Verification items for the finished model (mm, model axes). A direction names the side the tool comes from. Coordinates: 2 decimals unless noted, no trailing zeros. Write each loop counter-clockwise with the first axis right and the second up, starting at its lowest first coordinate (ties: lowest second). Pieces come first, ordered by that corner, then holes. Notation, with made-up numbers: (56.25, 10) - (60.25, 10) arc R23 ccw to (60.25, 22) - close; hole circle Ø2 at (35, 87). An arc over 180 degrees is marked (long way). Use one line per item in the form item = value. Start each with the question number.
(1) Tool access check on faces 1 (the cylindrical face through (-290.61, 3, 30.54)), 2 (the cylindrical face through (-283, 0, 7)), 3 (the flat face through (-3, 0, 42)), 4 (the flat face through (-290, 20.5, 21)). Record the directions out of +Z, -Z, +X, -X, +Y, -Y that give a thin tool (end or side, any length) a straight path to the whole face; none if there is none.
(2) Gauge pin test, flat ends, axial feed: pin 1 Ø5 at (x, y) = (-348.5, 14.5) entering from -Z; pin 2 Ø6 at (x, z) = (-383, 20.5) entering from -Y; pin 3 Ø6 at (x, z) = (-38.5, 31) entering from -Y. Record the tip position at first contact, or that the pin passes through.
(3) Mould release check, pull along Y, two halves, no side actions. Record for faces 5 (the cylindrical face through (-283, 0, 35)), 6 (the flat face through (-545, 10.2, 20.8)), 7 (the flat face through (-29, 0, 21)), 8 (the flat face through (-3, -21, 21)): released by +Y, released by -Y, zero draft, split by the parting line, or undercut.
(4) Sectioned sample at A-A (y = 0). Record the cut outline in (x, z), and give its area (3 significant figures).
(5) Material ranges on line 1 (Y direction, x = -67, z = 29); line 2 (Z direction, x = -509, y = 12.5); line 3 (Y direction, x = -13, z = 24), recorded low to high. Write a range as [from, to].
from build123d import *

# Parameters (mm, degrees)
SKETCH_1_W          = 516
SKETCH_1_H          = 35
SKETCH_1_W_2        = 5
SKETCH_1_H_2        = 42
SKETCH_1_W_3        = 48
EXTRUDE_1_DEPTH     = 42
SKETCH_3_W          = 516
SKETCH_3_H          = 42
CUT_EXTRUDE_1_DEPTH = 0.5
FILLET_1_R          = 7
SKETCH_4_R          = 10
CUT_EXTRUDE_2_DEPTH = 516
CUT_EXTRUDE_START   = -516
CUT_EXTRUDE_3_DEPTH = 516
FILLET_2_R          = 2
FILLET_3_R          = 4
FILLET_5_R          = 1
SKETCH_6_W          = 6.5
SKETCH_6_H          = 16
EXTRUDE_2_DEPTH     = 8


# Read off the part's stored shape, not the designer's step: Вырез-Вытянуть3
with BuildPart() as part:
    # Эскиз1 → Бобышка-Вытянуть1 (new body)
    with BuildSketch(Plane.XY):
        with Locations((-287, 3.5)):
            Rectangle(SKETCH_1_W, SKETCH_1_H)
        with Locations((-26.5, 0)):
            Rectangle(SKETCH_1_W_2, SKETCH_1_H_2)
        Rectangle(SKETCH_1_W_3, SKETCH_1_H_2)
    extrude(amount=EXTRUDE_1_DEPTH)

    # Эскиз3 → Вырез-Вытянуть1 (cut)
    with BuildSketch(Plane(origin=(0, 21, 0), x_dir=(1, 0, 0), z_dir=(0, 1, 0))):
        with Locations((-287, -21)):
            Rectangle(SKETCH_3_W, SKETCH_3_H)
    extrude(amount=-CUT_EXTRUDE_1_DEPTH, mode=Mode.SUBTRACT)

    # Скругление1
    fillet_1_edges = [part.edges().sort_by_distance(p)[0] for p in [
        (-287, -14, 42),
        (-287, -14, 0),
        (-287, 20.5, 0),
        (-287, 20.5, 42),
    ]]
    fillet(fillet_1_edges, radius=FILLET_1_R)

    # Эскиз4 → Вырез-Вытянуть2 (cut)
    with BuildSketch(Plane.ZY.offset(545)):
        with Locations((21, 0)):
            Circle(SKETCH_4_R)
    extrude(amount=-CUT_EXTRUDE_2_DEPTH, mode=Mode.SUBTRACT)

    # Вырез-Вытянуть3 outline → Вырез-Вытянуть3 (cut)
    with BuildSketch(Plane.ZY.offset(545).offset(CUT_EXTRUDE_START)):
        with BuildLine():
            ThreePointArc((11.715680056, -10.478616473), (8.035714286, -10.206727973), (8.63508525, -6.565735543))
            ThreePointArc((8.63508525, -6.565735543), (7, 0), (8.63508525, 6.565735543))
            ThreePointArc((8.63508525, 6.565735543), (7.60351338, 9.372189345), (10, 11.160254038))
            Line((10, 11.160254038), (10, 20.5))
            Line((10, 20.5), (7, 20.5))
            ThreePointArc((7, 20.5), (2.050252532, 18.449747468), (0, 13.5))
            Line((0, 13.5), (0, -7))
            ThreePointArc((0, -7), (2.050252532, -11.949747468), (7, -14))
            Line((7, -14), (21.000000051, -14))
            ThreePointArc((21.000000051, -14), (16.035155143, -13.090084627), (11.715680056, -10.478616473))
        make_face()
        with BuildLine():
            ThreePointArc((30.284319944, -10.478616473), (25.964844905, -13.090084609), (21.000000051, -14))
            Line((21.000000051, -14), (35, -14))
            ThreePointArc((35, -14), (39.949747468, -11.949747468), (42, -7))
            Line((42, -7), (42, 13.5))
            ThreePointArc((42, 13.5), (39.949747468, 18.449747468), (35, 20.5))
            Line((35, 20.5), (32, 20.5))
            Line((32, 20.5), (32, 11.160254038))
            ThreePointArc((32, 11.160254038), (34.39648662, 9.372189345), (33.36491475, 6.565735543))
            ThreePointArc((33.36491475, 6.565735543), (35, 0), (33.36491475, -6.565735543))
            ThreePointArc((33.36491475, -6.565735543), (33.964285714, -10.206727973), (30.284319944, -10.478616473))
        make_face()
    extrude(amount=CUT_EXTRUDE_3_DEPTH, mode=Mode.SUBTRACT)

    # Скругление2
    fillet_2_edges = [part.edges().sort_by_distance(p)[0] for p in [
        (-287, 20.5, 10),
        (-287, 20.5, 32),
    ]]
    fillet(fillet_2_edges, radius=FILLET_2_R)

    # Скругление3
    fillet_3_edges = [part.edges().sort_by_distance(p)[0] for p in [
        (-2.5, -21, 42),
        (-2.5, 21, 42),
        (-2.5, 21, 0),
        (-2.5, -21, 0),
    ]]
    fillet(fillet_3_edges, radius=FILLET_3_R)

    # Скругление5
    fillet_5_edges = [part.edges().sort_by_distance(p)[0] for p in [
        (-287, 11.160254038, 10),
        (-545, 9.372189345, 7.60351338),
        (-287, 6.565735543, 8.63508525),
        (-545, 0, 7),
        (-545, 14.830127019, 10),
        (-287, 6.565735543, 33.36491475),
        (-545, 9.372189345, 34.39648662),
        (-287, 11.160254038, 32),
        (-545, 14.830127019, 32),
        (-287, -10.478616473, 30.284319944),
        (-545, -10.206727973, 33.964285714),
        (-287, -6.565735543, 33.36491475),
        (-545, 0, 35),
        (-545, 20.5, 21),
        (-545, 19.914213562, 31.414213562),
        (-545, 19.914213562, 10.585786438),
        (-287, -6.565735543, 8.63508525),
        (-545, -10.206727973, 8.035714286),
        (-287, -10.478616473, 11.715680056),
        (-545, -13.090084627, 16.035155143),
    ]]
    fillet(fillet_5_edges, radius=FILLET_5_R)

    # Эскиз6 → Бобышка-Вытянуть2 (add)
    with BuildSketch(Plane(origin=(0, 21, 0), x_dir=(1, 0, 0), z_dir=(0, 1, 0))):
        with Locations((20.75, -21)):
            Rectangle(SKETCH_6_W, SKETCH_6_H)
    extrude(amount=EXTRUDE_2_DEPTH)


solid = part.part
Answers below:
q1.face_1 = -X
q1.face_2 = -Z, -X
q1.face_3 = +Z, +X, -X, +Y, -Y
q1.face_4 = +Z, -Z, -X, +Y
q2.pin_1 = 10
q2.pin_2 = -14
q2.pin_3 = -12.12
q3.face_5 = undercut
q3.face_6 = zero draft
q3.face_7 = undercut
q3.face_8 = released by -Y
q4.outline = (-545, 8) arc R1 ccw to (-544, 7) - (-29, 7) - (-29, 0) - (24, 0) - (24, 42) - (-29, 42) - (-29, 35) - (-544, 35) arc R1 ccw to (-545, 34) - (-545, 31) - (-29, 31) - (-29, 11) - (-545, 11) - close
q4.area = 6,350 mm2
q5.line_1 = [-11.49, -6], [6, 20.5]
q5.line_2 = [10, 32]
q5.line_3 = [-21, 21]
